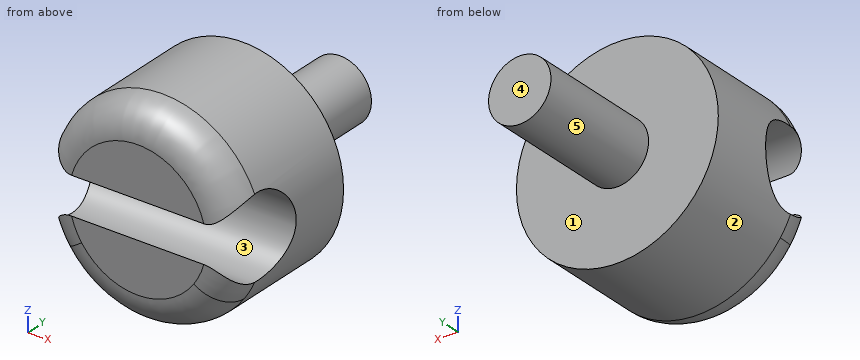
```python
from build123d import *

# Parameters (mm, degrees)
F0_R        = 31.2849976613
F1_DEPTH    = 43
F2_R        = 12.5
F3_DEPTH    = 40
F4_T3_ANGLE = 250.4726360275
F4_T6_ANGLE = 250.4726360275
F5_R        = 9.6724066991
F6_DEPTH    = 40


# Not quite as in the source:
# - a fillet or chamfer that OpenCascade refuses, or shapes differently, is made with other operations: its cross-section is extruded or revolved along the edge and cut away or added


with BuildPart() as f1:
    # F0 (on Front) → F1 (new body)
    with BuildSketch(Plane.XZ):
        with Locations((3.0078960117, 0)):
            Circle(F0_R)
    extrude(amount=F1_DEPTH)

    # F2 (on Right) → F3 (cut, symmetric)
    with BuildSketch(Plane.YZ):
        with Locations((-31.9053208832, 0)):
            Circle(F2_R)
    extrude(amount=F3_DEPTH, both=True, mode=Mode.SUBTRACT)

    # F4: fillet of radius 10 on 2 edges, made by hand


with BuildPart() as f4_tool1:
    # F4_s2 → F4_t3 (revolve)
    with BuildSketch(Plane(origin=(1.0012428292, 0, 1.4174438647), x_dir=(0, 1, 0), z_dir=(-0.5769501631, 0, -0.8167793517))):
        with BuildLine():
            ThreePointArc((-33, 33.7417850156), (-40.0710678119, 30.8128528275), (-43, 23.7417850156))
            Line((-43, 23.7417850156), (-43, 33.7417850156))
            Line((-43, 33.7417850156), (-33, 33.7417850156))
        make_face()
    revolve(axis=Axis((3.0078960117, -43, 0), (0, -1, 0)), revolution_arc=F4_T3_ANGLE)


with BuildPart() as f4_tool4:
    # F4_s5 → F4_t6 (revolve)
    with BuildSketch(Plane(origin=(1.0012428292, 0, 1.4174438647), x_dir=(0, 1, 0), z_dir=(0.5769501631, 0, 0.8167793517))):
        with BuildLine():
            ThreePointArc((-33, 28.828210307), (-40.0710678119, 25.8992781188), (-43, 18.828210307))
            Line((-43, 18.828210307), (-43, 28.828210307))
            Line((-43, 28.828210307), (-33, 28.828210307))
        make_face()
    revolve(axis=Axis((3.0078960117, -43, 0), (0, -1, 0)), revolution_arc=F4_T6_ANGLE)


with BuildPart() as f1_1:
    add(f1.part)

    # F4_t7: cut F4_tool1, F4_tool4
    add([f4_tool1.part, f4_tool4.part], mode=Mode.SUBTRACT)

    # F5 (on face) → F6 (join)
    with BuildSketch(Plane(origin=(0, 0, 0), x_dir=(-1, 0, 0), z_dir=(0, 1, 0))):
        with Locations((-3.0078960117, 0)):
            Circle(F5_R)
    extrude(amount=F6_DEPTH)


solid = f1_1.part
```
Check sheet for the modelled part. Datum: model origin and axes. Units: mm. Face numbers are marked on the shaded views. A direction names the side the tool comes from. Coordinates: 2 decimals unless noted, no trailing zeros. Write each loop counter-clockwise with the first axis right and the second up, starting at its lowest first coordinate (ties: lowest second). Pieces come first, ordered by that corner, then holes. Notation, with made-up numbers: M 7.25,13.25 L 37.25,13.25 A18 ccw 37.25,33.25 Z; hole C 14,15 d5. An arc over 180 degrees is marked long. Write item = value, one per line. Start each with the question number.
1. Tool access check on the marked faces 4 and 5. Record the directions out of +Z, -Z, +X, -X, +Y, -Y that give a thin tool (end or side, any length) a straight path to the whole face; none if there is none.
2. Sectioned sample at D-D (y = -6.5). Record the cut outline in (x, z) (3 decimals), then the cut area to 3 significant figures.
3. Sectioned sample at B-B (y = 11). Record the cut outline in (x, z), then the cut area to 3 significant figures.
4. Sectioned sample at C-C (y = -24.5). Record the cut outline in (x, z) (3 decimals), then the cut area to 3 significant figures.
5. Sectioned sample at A-A (z = 0). Record the cut outline in (x, y).
6. Go/stop test with flat-tipped pins: pin 1 (3 mm diameter, centred on x = -11, y = -31.5, fed in from +Z); pin 2 (12 mm diameter, centred on y = 0, z = 9, fed in from -X); pin 3 (3 mm diameter, centred on x = -15, z = -16.5, fed in from -Y). Record where each tip stops, or that it passes through.
7. Mould release check, pull along Z, two halves, no side actions. Record for the marked faces 1, 2 and 3: pulls with the +Z half, pulls with the -Z half, needs draft (parallel to the pull), parting line crosses it, or undercut.
8. Thickness scan on probe 1 along Y at (x, z) = (-11.5, 0); probe 2 along Y at (x, z) = (4, 0); probe 3 along Y at (x, z) = (-22, -8). Record the ranges inside material, lowest first.
The answers:
q1.face_4 = +Z, -Z, +X, -X, +Y
q1.face_5 = +Y
q2.outline = C 3.008,0 d62.57
q2.area = 3,070 mm²
q3.outline = C 3.01,0 d19.34
q3.area = 294 mm²
q4.outline = M -26.612,-10.07 A31.285 ccw 32.628,-10.07 Z; M -26.612,10.07 L 32.628,10.07 A31.285 ccw Z
q4.area = 1,840 mm²
q5.outline = M -28.28,-19.41 L 34.29,-19.41 L 34.29,0 L 12.68,0 L 12.68,40 L -6.66,40 L -6.66,0 L -28.28,0 Z
q6.pin_1 = 28.68
q6.pin_2 = -28.13
q6.pin_3 = -42.86
q7.face_1 = needs draft
q7.face_2 = parting line crosses it
q7.face_3 = undercut
q8.probe_1 = -19.41 to 0
q8.probe_2 = -19.41 to 40
q8.probe_3 = -41.68 to -41.51, -22.3 to 0
